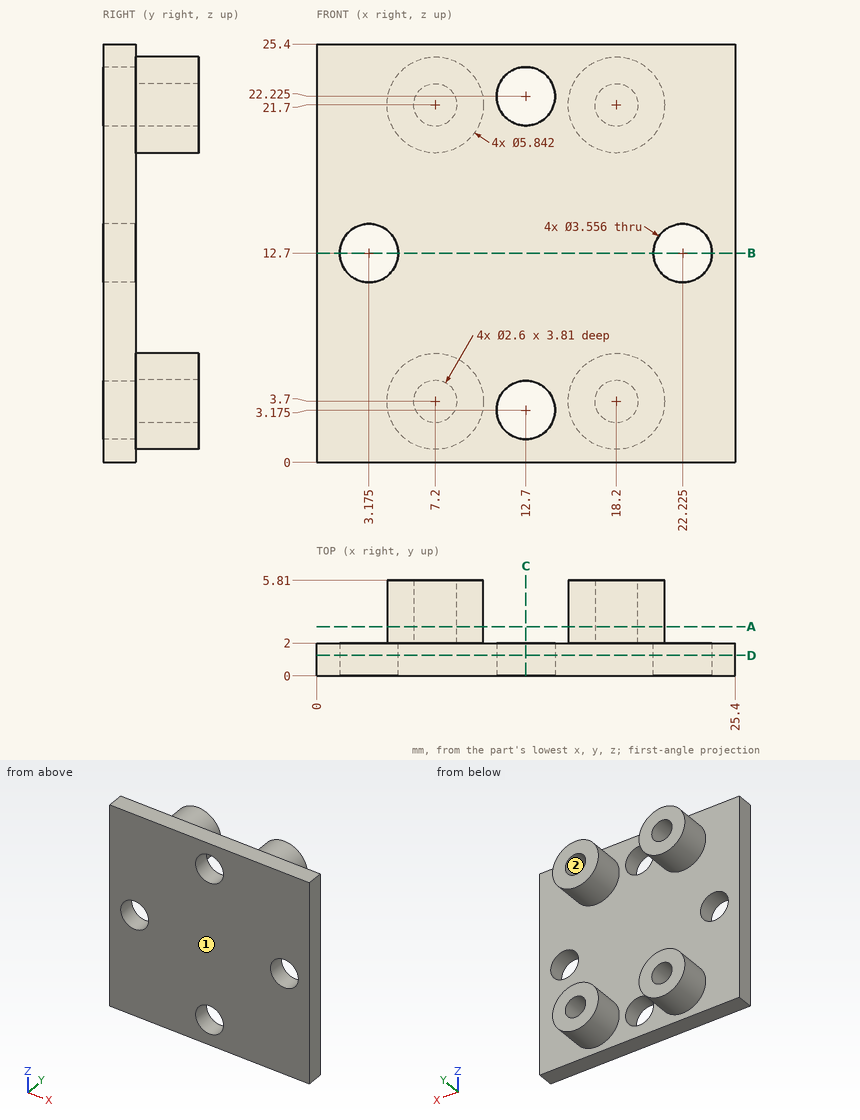
Check sheet for the drawn part. Datum: minimum x, y, z corner. Units: mm. Round coordinates to 2 decimals unless told otherwise and drop trailing zeros. Write each loop counter-clockwise with the first axis right and the second up, starting at its lowest first coordinate (ties: lowest second). Pieces come first, ordered by that corner, then holes. Notation, with made-up numbers: (-20, -34) -> (12, -34) arc R20 ccw to (12, -20) -> close; hole circle Ø8 at (4, -17.5). An arc over 180 degrees is marked (long way). One line per item, written item: value. Start each with the question number.
(1) Scan lines: line 1 (Z direction, x = 18.2, y = 3.5); line 2 (Z direction, x = 12.75, y = 1.25); line 3 (X direction, y = 3.05, z = 3.7). Record each from-to range of solid material in increasing order. Write a range as [from, to].
(2) Cross-section at D-D, the plane y = 1.25. Record the cut outline in (x, z) (3 decimals).
(3) Go/stop test with flat-tipped pins: pin 1 Ø0.8 at (x, z) = (18, 21.5) entering from +Y; pin 2 Ø3 at (x, y) = (9, 4) entering from +Z; pin 3 Ø1 at (x, y) = (17.5, 5) entering from -Z. Record where each tip stops, or that it passes through.
(4) Cross-section at B-B, the plane z = 12.7. Record the cut outline in (x, y).
(5) Draft check along X on the marked faces 1 and 2. Enter one of: +X half, -X half, draft (parallel to the pull), parting line (faces both ways), or undercut.
(6) Cross-section at A-A, the plane y = 3. Record the cut outline in (x, z), and give its area (3 significant figures).
(7) Cross-section at C-C, the plane x = 12.7. Record the cut outline in (y, z).
Answer:
1. line 1: [0.78, 2.4], [5, 6.62], [18.78, 20.4], [23, 24.62]
1. line 2: [0, 1.4], [4.95, 20.45], [24, 25.4]
1. line 3: [4.28, 5.9], [8.5, 10.12], [15.28, 16.9], [19.5, 21.12]
2. outline: (0, 0) -> (25.4, 0) -> (25.4, 25.4) -> (0, 25.4) -> close; hole circle Ø3.556 at (3.175, 12.7); hole circle Ø3.556 at (12.7, 3.175); hole circle Ø3.556 at (12.7, 22.225); hole circle Ø3.556 at (22.225, 12.7)
3. pin 1: y = 2
3. pin 2: z = 24.61
3. pin 3: z = 0.79
4. outline: (0, 0) -> (1.4, 0) -> (1.4, 2) -> (0, 2) -> close; (4.95, 0) -> (20.45, 0) -> (20.45, 2) -> (4.95, 2) -> close; (24, 0) -> (25.4, 0) -> (25.4, 2) -> (24, 2) -> close
5. face 1: draft
5. face 2: undercut
6. outline: circle Ø5.84 at (7.2, 3.7); circle Ø5.84 at (7.2, 21.7); circle Ø5.84 at (18.2, 3.7); circle Ø5.84 at (18.2, 21.7); hole circle Ø2.6 at (7.2, 3.7); hole circle Ø2.6 at (7.2, 21.7); hole circle Ø2.6 at (18.2, 3.7); hole circle Ø2.6 at (18.2, 21.7)
6. area: 86.0 mm²
7. outline: (0, 0) -> (2, 0) -> (2, 1.4) -> (0, 1.4) -> close; (0, 4.95) -> (2, 4.95) -> (2, 20.45) -> (0, 20.45) -> close; (0, 24) -> (2, 24) -> (2, 25.4) -> (0, 25.4) -> close
